Input: part model. Units: mm. Frame: model coordinates. Round coordinates to 2 decimals unless told otherwise and drop trailing zeros. Order: outer loops, then holes, each group sorted by start corner. A loop starts at its lowest first (then second) coordinate and runs counter-clockwise, first axis right, second up. Notation, with made-up numbers: (59.5, 82.5) - (94.5, 82.5) arc R24 ccw to (94.5, 105.5) - close; hole circle Ø6 at (24.5, 58.25). An arc over 180 degrees is marked (long way). One line per item, written item: value. Start each with the question number.
Autodesk Inventor part; units mm, degrees
ref_plane "YZ Plane" through (0, 0, 0) normal (1, 0, 0) x (0, 1, 0)
ref_plane "XZ Plane" through (0, 0, 0) normal (0, 1, 0) x (-1, 0, 0)
ref_plane "XY Plane" through (0, 0, 0) normal (0, 0, 1) x (1, 0, 0)
sketch "Sketch1" plane through (-41.0022, 83.9754, 0) normal (0, 0, 1) x (1, 0, 0)
  line L0 (43.6907, -84.1601) -> (79.4807, -84.1601)
  arc A0 (43.6907, -84.1601) -> (41.6657, -84.1611) centre (42.6783, -84.1982) ccw
  line L1 (-40.3343, -84.1601) -> (41.6657, -84.1611)
  arc A1 (-40.3343, -84.1601) -> (-42.3343, -84.1611) centre (-41.3342, -84.1854) ccw
  line L2 (-78.1393, -84.1601) -> (-42.3343, -84.1611)
  arc A2 (-83.3093, -78.9901) -> (-78.1393, -84.1601) centre (-78.1401, -78.9909) ccw
  line L3 (-83.3093, -43.2101) -> (-83.3093, -78.9901)
  arc A3 (-83.3093, -43.2101) -> (-83.3103, -41.1851) centre (-83.3474, -42.1976) ccw
  line L4 (-83.3093, 40.8149) -> (-83.3103, -41.1851)
  arc A4 (-83.3093, 40.8149) -> (-83.3103, 42.8149) centre (-83.3346, 41.8149) ccw
  line L5 (-83.3093, 78.6259) -> (-83.3103, 42.8149)
  arc A5 (-78.1463, 83.7899) -> (-83.3093, 78.6259) centre (-78.147, 78.6276) ccw
  line L6 (-42.3343, 83.7899) -> (-78.1463, 83.7899)
  arc A6 (-42.3343, 83.7899) -> (-40.3343, 83.7899) centre (-41.3343, 83.8153) ccw
  line L7 (41.6657, 83.7899) -> (-40.3343, 83.7899)
  arc A7 (41.6657, 83.7899) -> (43.6657, 83.7909) centre (42.6657, 83.8152) ccw
  line L8 (79.4797, 83.7899) -> (43.6657, 83.7909)
  arc A8 (84.6457, 78.6229) -> (79.4797, 83.7899) centre (79.48, 78.6242) ccw
  line L9 (84.6457, 42.8349) -> (84.6457, 78.6229)
  arc A9 (84.6457, 42.8349) -> (84.6417, 40.8149) centre (84.6762, 41.8249) ccw
  line L10 (84.6407, -41.1851) -> (84.6417, 40.8149)
  arc A10 (84.6407, -41.1851) -> (84.6417, -43.1851) centre (84.666, -42.1851) ccw
  line L11 (84.6407, -79.0001) -> (84.6417, -43.1851)
  arc A11 (79.4807, -84.1601) -> (84.6407, -79.0001) centre (79.4819, -79.0012) ccw
  circle A12 centre (42.6657, 73.3149) radius 1
  circle A13 centre (-41.3343, 73.3149) radius 1
  circle A14 centre (-41.3343, -73.6851) radius 1
  circle A15 centre (42.6657, -73.6851) radius 1
  circle A16 centre (74.1657, -0.1851) radius 1
  line L12 (15.5981, 38.5892) -> (-36.6892, 38.5892)
  line L13 (-36.6892, 38.5892) -> (-36.6892, 44.7944)
  line L14 (-36.6892, 44.7944) -> (15.5981, 44.7944)
  line L15 (15.5981, 44.7944) -> (15.5981, 38.5892)
  line L16 (15.5981, -45.4168) -> (-36.6892, -45.4168)
  line L17 (-36.6892, -45.4168) -> (-36.6892, -39.2116)
  line L18 (-36.6892, -39.2116) -> (15.5981, -39.2116)
  line L19 (15.5981, -39.2116) -> (15.5981, -45.4168)
  point P0 (0.6657, -0.1851)
  point P1 (-10.5892, -42.205)
  point P2 (-10.5892, 41.801)
  point P3 (-10.5892, -42.205)
extrude "Extrusion1" add sketch "Sketch1" along normal blind 3
properties part number "PCB Protector for Small Board" material "Glass"
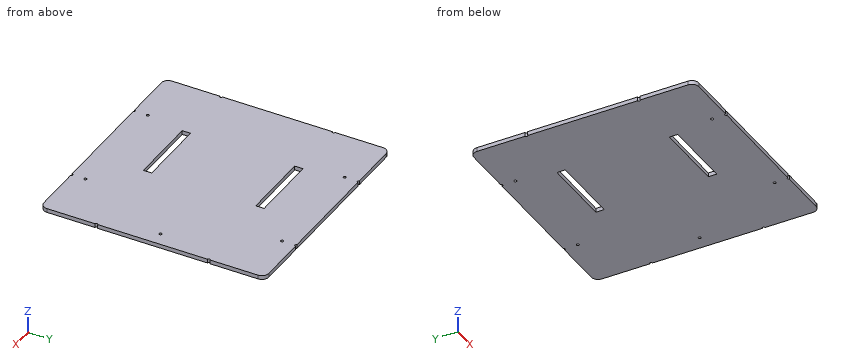
1. Section C-C (z = 1.3). State how many separate pieces and enclosed holes the cut face has, then the cut area to 3 significant figures.
2. Section A-A (x = -34). Return the cut outline in (y, z).
3. Pin query (flat end, axial travel): pin 1 (0.9 mm diameter, centred on y = 30.5, z = 1.5, fed in from +X); pin 2 (2.5 mm diameter, centred on x = -82.34, y = 10.29, fed in from +Z). Return the tip coordinate at first contact, or that it passes through.
4. Section B-B (x = -73). Return the cut outline in (y, z), then the cut area to 3 significant figures.
5. Line query: line 1 (Y direction, x = -50.5, z = 1.4); line 2 (X direction, y = 39.5, z = 2.65); line 3 (Y direction, x = 8.5, z = 1.65). Output: solid intervals per line, ascending. Write a range as from..to.
Solved:
1. separate pieces: 1
1. enclosed holes: 7
1. area: 27,500 mm²
2. outline: (-0.19, 0) - (38.56, 0) - (38.56, 3) - (-0.19, 3) - close; (44.76, 0) - (122.56, 0) - (122.56, 3) - (44.76, 3) - close; (128.77, 0) - (167.77, 0) - (167.77, 3) - (128.77, 3) - close
3. pin 1: stops at x = 43.64
3. pin 2: stops at z = 3
4. outline: (-0.18, 0) - (38.56, 0) - (38.56, 3) - (-0.18, 3) - close; (44.76, 0) - (122.56, 0) - (122.56, 3) - (44.76, 3) - close; (128.77, 0) - (167.77, 0) - (167.77, 3) - (128.77, 3) - close
4. area: 467 mm²
5. line 1: y = -0.19..38.56, 44.76..122.56, 128.77..167.77
5. line 2: x = -124.31..-77.69, -25.4..43.64
5. line 3: y = -0.18..167.77
